Read the model definition and answer for the solid it produces. Units are mm, in the model's axes. Face numbers are marked on the shaded views. A direction names the side the tool comes from. Coordinates: 2 decimals unless noted, no trailing zeros. Write each loop counter-clockwise with the first axis right and the second up, starting at its lowest first coordinate (ties: lowest second). Pieces come first, ordered by that corner, then holes. Notation, with made-up numbers: (-4.5, -35.5) - (48.5, -35.5) arc R15 ccw to (48.5, -18.5) - close; hole circle Ø10 at (89.25, 66.25). An arc over 180 degrees is marked (long way). Return JSON: item names as keys, results as strings.
Autodesk Inventor part; units mm, degrees
ref_plane "YZ Plane" through (0, 0, 0) normal (1, 0, 0) x (0, 1, 0)
ref_plane "XZ Plane" through (0, 0, 0) normal (0, 1, 0) x (-1, 0, 0)
ref_plane "XY Plane" through (0, 0, 0) normal (0, 0, 1) x (1, 0, 0)
sketch "Boceto1" plane through (0, 0, 0) normal (0, 0, 1) x (1, 0, 0)
  line L0 (-58.5, -19) -> (58.5, -19)
  line L1 (63.5, -14) -> (63.5, 14)
  line L2 (58.5, 19) -> (-58.5, 19)
  line L3 (-63.5, 14) -> (-63.5, -14)
  line L4 (-63.5, -19) -> (63.5, 19) construction
  line L5 (63.5, -19) -> (-63.5, 19) construction
  arc A0 (-58.5, 19) -> (-63.5, 14) centre (-58.5, 14) ccw
  arc A1 (-63.5, -14) -> (-58.5, -19) centre (-58.5, -14) ccw
  arc A2 (58.5, -19) -> (63.5, -14) centre (58.5, -14) ccw
  arc A3 (63.5, 14) -> (58.5, 19) centre (58.5, 14) ccw
  line L6 (-63.5, 0) -> (63.5, 0) construction
  line L7 (-58.5, 0) -> (-39.5, 0) construction
  line L8 (-52, -6.5) -> (-46, -6.5)
  line L9 (-46, 6.5) -> (-52, 6.5)
  arc A4 (-52, 6.5) -> (-52, -6.5) centre (-52, 0) ccw
  arc A5 (-46, -6.5) -> (-46, 6.5) centre (-46, 0) ccw
  line L10 (0, 19) -> (0, -19) construction
  line L11 (52, -6.5) -> (46, -6.5)
  line L12 (46, 6.5) -> (52, 6.5)
  arc A6 (52, -6.5) -> (52, 6.5) centre (52, 0) ccw
  arc A7 (46, 6.5) -> (46, -6.5) centre (46, 0) ccw
  point P0 (0, 0)
  point P1 (-49, 0)
  dimension "d0" = 38
  dimension "d1" = 127
  dimension "d2" = 5
  dimension "d3" = 5
  dimension "d4" = 19
  dimension "d6" = 13
extrude "Extrusión1" add sketch "Boceto1" along normal blind 20
properties part number "SoporteMancal"
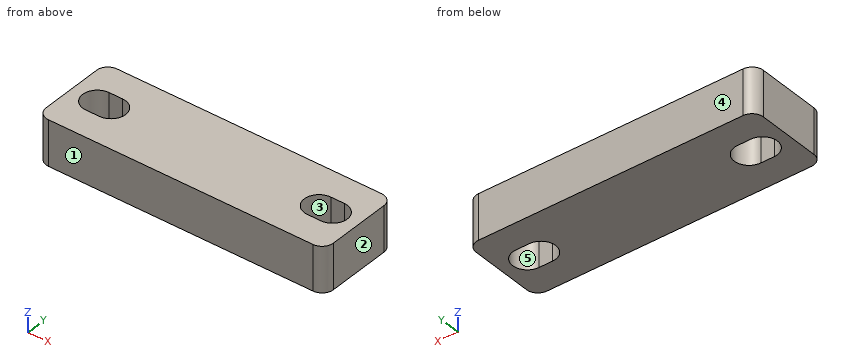
(1) A cutting plane is placed at D-D (x = -42). Determine the outline of the cut face in (y, z), and give its area (3 significant figures).
Answer:
{"outline": "(-19, 0) - (-5.12, 0) - (-5.12, 20) - (-19, 20) - close; (5.12, 0) - (19, 0) - (19, 20) - (5.12, 20) - close", "area": "555 mm²"}
(2) Straight lines are drawn through the part: line 1 (X direction, y = 3, z = 6.25); line 2 (X direction, y = 2, z = 18.75); line 3 (Y direction, x = 46, z = 10.75). For each, find the intervals that lie inside material, in ascending order. Write a range as from..to.
Answer:
{"line 1": "-63.5..-57.77, -40.23..40.23, 57.77..63.5", "line 2": "-63.5..-58.18, -39.82..39.82, 58.18..63.5", "line 3": "-19..-6.5, 6.5..19"}
(3) A cutting plane is placed at B-B (y = 0). Determine the outline of the cut face in (x, z), and give its area (3 significant figures).
Answer:
{"outline": "(-63.5, 0) - (-58.5, 0) - (-58.5, 20) - (-63.5, 20) - close; (-39.5, 0) - (39.5, 0) - (39.5, 20) - (-39.5, 20) - close; (58.5, 0) - (63.5, 0) - (63.5, 20) - (58.5, 20) - close", "area": "1,780 mm²"}
(4) Determine the mould class of the marked faces 1, 2 and 3 for opening direction X: +X half, -X half, draft (parallel to the pull), parting line (faces both ways), or undercut.
Answer:
{"face 1": "draft", "face 2": "+X half", "face 3": "undercut"}
(5) A cutting plane is placed at A-A (z = 17.5). Determine the outline of the cut face in (x, y).
Answer:
{"outline": "(-63.5, -14) arc R5 ccw to (-58.5, -19) - (58.5, -19) arc R5 ccw to (63.5, -14) - (63.5, 14) arc R5 ccw to (58.5, 19) - (-58.5, 19) arc R5 ccw to (-63.5, 14) - close; hole (-52, -6.5) - (-46, -6.5) arc R6.5 ccw to (-46, 6.5) - (-52, 6.5) arc R6.5 ccw to start; hole (46, -6.5) - (52, -6.5) arc R6.5 ccw to (52, 6.5) - (46, 6.5) arc R6.5 ccw to start"}
(6) A cutting plane is placed at C-C (x = 53.5). Determine the outline of the cut face in (y, z), and give its area (3 significant figures).
Answer:
{"outline": "(-19, 0) - (-6.32, 0) - (-6.32, 20) - (-19, 20) - close; (6.32, 0) - (19, 0) - (19, 20) - (6.32, 20) - close", "area": "507 mm²"}
(7) Which of the six approach directions +Z, -Z, +X, -X, +Y, -Y give full straight-line access (tool end or side, diameter ignored) to the marked faces 4 and 5?
Answer:
{"face 4": "+Z, -Z, +X, -X, +Y", "face 5": "+Z, -Z"}
